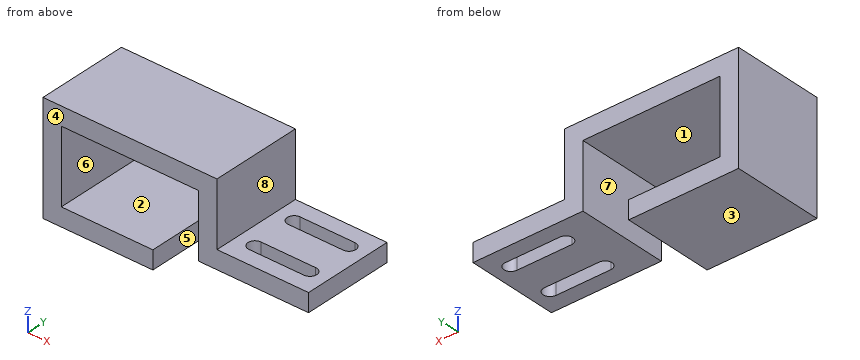
from build123d import *

# Parameters (mm, degrees)
SALIENTE_EXTRUIR1_DEPTH = 20
CORTAR_EXTRUIR1_DEPTH   = 20
CROQUIS3_W              = 4
CROQUIS3_H              = 20
SALIENTE_EXTRUIR2_DEPTH = 20


with BuildPart() as part:
    # Croquis1 → Saliente-Extruir1 (new body)
    with BuildSketch(Plane(origin=(0, 0, 0), x_dir=(1, 0, 0), z_dir=(0, 1, 0))):
        Polygon((-19, 24), (-15, 24), (-15, 4), (15, 4), (15, 18), (39, 18), (39, 14), (19, 14), (19, 0), (-19, 0), align=None)
    extrude(amount=SALIENTE_EXTRUIR1_DEPTH)

    # Croquis2 → Cortar-Extruir1 (cut)
    with BuildSketch(Plane.XY.offset(-14)):
        with BuildLine():
            Line((35, 16.5), (23, 16.5))
            ThreePointArc((23, 16.5), (21.5, 15), (23, 13.5))
            Line((23, 13.5), (35, 13.5))
            ThreePointArc((35, 13.5), (36.5, 15), (35, 16.5))
        make_face()
        with BuildLine():
            Line((35, 3.5), (23, 3.5))
            ThreePointArc((23, 3.5), (21.5, 5), (23, 6.5))
            Line((23, 6.5), (35, 6.5))
            ThreePointArc((35, 6.5), (36.5, 5), (35, 3.5))
        make_face()
    extrude(amount=-CORTAR_EXTRUIR1_DEPTH, mode=Mode.SUBTRACT)

    # Croquis3 → Saliente-Extruir2 (add)
    with BuildSketch(Plane(origin=(-15, 0, 0), x_dir=(0, 0, -1), z_dir=(1, 0, 0))):
        with Locations((22, 10)):
            Rectangle(CROQUIS3_W, CROQUIS3_H)
    extrude(amount=SALIENTE_EXTRUIR2_DEPTH)


solid = part.part
Could you check a few things on this model? Use its own coordinates, in mm. Face numbers are marked on the shaded views. A direction names the side the tool comes from. Give positions to 0.01 mm unless a question says otherwise; leave off trailing zeros. Order: outer loops, then holes, each group sorted by start corner. A loop starts at its lowest first (then second) coordinate and runs counter-clockwise, first axis right, second up. Notation, with made-up numbers: (8, 30) - (37, 30) arc R18 cw to (37, 35) - close; hole circle Ø5 at (84.25, 86.25). An arc over 180 degrees is marked (long way). One line per question, with ' | ' between items. Start each with the question number.
Item 1: I need wall thicknesses on probe 1 along X at (y, z) = (6.5, -5); probe 2 along Z at (x, y) = (2, 12); probe 3 along X at (y, z) = (15.5, -14.25). Which ranges of each line are inside material? Lowest first, please. Write a range as [from, to].
Item 2: I want a section at A-A on z = -16.75. Write out the boundary of the cut face in (x, y), then the cut area to 3 significant figures.
Item 3: I want a section at C-C on z = -4.75. Write out the boundary of the cut face in (x, y), then the cut area to 3 significant figures.
Item 4: Thinking about a two-plate mould opening in Z: for the marked faces 1, 2, 3 and 4, which applies, pulls with the +Z half, pulls with the -Z half, needs draft (parallel to the pull), parting line crosses it, or undercut?
Item 5: I want a section at B-B on y = 15. Write out the boundary of the cut face in (x, z), then the cut area to 3 significant figures.
Item 6: I'm going to push flat-ended pins straight in: pin 1 Ø6 at (x, y) = (21.5, 6.5) entering from -Z; pin 2 Ø2 at (y, z) = (10.5, -22.5) entering from +X; pin 3 Ø1 at (y, z) = (8, -6.5) entering from +X. Where does each tip first touch, or does it pass through?
Item 7: I want a section at D-D on y = 10.5. Write out the boundary of the cut face in (x, z).
Item 8: For the marked faces 5, 6, 7 and 8, which set-ups out of +Z, -Z, +X, -X, +Y, -Y let a thin tool reach every point of the face, with its end or its side?
Verdict:
1) probe 1: [-19, -15], [15, 19] | probe 2: [-24, -20], [-4, 0] | probe 3: [-19, -15], [15, 21.59], [36.41, 39]
2) outline: (-19, 0) - (-15, 0) - (-15, 20) - (-19, 20) - close; (15, 0) - (39, 0) - (39, 20) - (15, 20) - close; hole (23, 3.5) - (35, 3.5) arc R1.5 ccw to (35, 6.5) - (23, 6.5) arc R1.5 ccw to start; hole (23, 13.5) - (35, 13.5) arc R1.5 ccw to (35, 16.5) - (23, 16.5) arc R1.5 ccw to start | area: 474 mm^2
3) outline: (-19, 0) - (-15, 0) - (-15, 20) - (-19, 20) - close; (15, 0) - (19, 0) - (19, 20) - (15, 20) - close | area: 160 mm^2
4) face 1: undercut | face 2: undercut | face 3: pulls with the -Z half | face 4: needs draft
5) outline: (-19, -24) - (5, -24) - (5, -20) - (-15, -20) - (-15, -4) - (15, -4) - (15, -18) - (21.5, -18) - (21.5, -14) - (19, -14) - (19, 0) - (-19, 0) - close; (36.5, -18) - (39, -18) - (39, -14) - (36.5, -14) - close | area: 388 mm^2
6) pin 1: z = -18 | pin 2: x = 5 | pin 3: x = 19
7) outline: (-19, -24) - (5, -24) - (5, -20) - (-15, -20) - (-15, -4) - (15, -4) - (15, -18) - (39, -18) - (39, -14) - (19, -14) - (19, 0) - (-19, 0) - close
8) face 5: -Z, +X, +Y, -Y | face 6: +Y, -Y | face 7: -Z, +Y, -Y | face 8: +Z, +X, +Y, -Y
